The model under review builds one solid part; all positions refer to its coordinate system, in mm. A direction names the side the tool comes from. Round coordinates to 2 decimals unless told otherwise and drop trailing zeros. Write each loop counter-clockwise with the first axis right and the second up, starting at its lowest first coordinate (ties: lowest second). Pieces come first, ordered by that corner, then holes. Notation, with made-up numbers: (40.5, 66.5) -> (90.5, 66.5) arc R25 cw to (90.5, 100.5) -> close; hole circle Ø10 at (9.25, 9). An arc over 180 degrees is marked (long way). Answer in a Markdown table with one row per item. Add a question column.
```python
from build123d import *

# Parameters (mm, degrees)
SKETCH1_W           = 190.5
SKETCH1_H           = 6.35
BOSS_EXTRUDE1_DEPTH = 3.175
BOSS_EXTRUDE2_DEPTH = 3.175
LPATTERN1_COUNT     = 62
LPATTERN1_PITCH     = 2.54


with BuildPart() as part:
    # Sketch1 → Boss-Extrude1 (new body)
    with BuildSketch(Plane.XY):
        with Locations((95.25, 3.175)):
            Rectangle(SKETCH1_W, SKETCH1_H)
    extrude(amount=BOSS_EXTRUDE1_DEPTH)

    # Sketch2 → Boss-Extrude2 (add)
    with BuildSketch(Plane.XY.offset(3.175)):
        Polygon((165.1, 6.35), (163.83, 8.89), (162.56, 6.35), align=None)
    boss_extrude2 = extrude(amount=-BOSS_EXTRUDE2_DEPTH)

    # LPattern1: Boss-Extrude2 ×62
    with Locations(*[(-i * LPATTERN1_PITCH, 0, 0) for i in range(1, LPATTERN1_COUNT)]):
        add(boss_extrude2)


solid = part.part
```
1. Insertion check: pin 1 Ø1.5 at (x, z) = (46, 1.5) entering from +Y. The pin has a flat end and moves straight along its axis. Give the tip position at first contact, or say it passes through.
2. Tool access review of faces 1 (the flat face through (178, 6.35, 2)), 2 (the flat face through (94, 4, 0)), 3 (the flat face through (4, 6.35, 2)): name each direction out of +Z, -Z, +X, -X, +Y, -Y from which nothing blocks a thin tool from reaching the whole face with its end or side.
3. For L1, parallel to Y at x = 176.5, z = 0.9; L2, parallel to Y at x = 18.5, z = 2.85, list the stretches that pass through material, from the lowest coordinate up.
4. Add section A-A on x = 175.5. Write out the cut boundary in (y, z) (3 decimals).
Filled in:
| question | item | result |
|---|---|---|
| 1 | pin 1 | y = 8.41 |
| 2 | face 1 | +Z, -Z, +X, +Y |
| 2 | face 2 | -Z, +X, -X, +Y, -Y |
| 2 | face 3 | +Z, -Z, -X, +Y |
| 3 | L1 | 0 to 6.35 |
| 3 | L2 | 0 to 7.79 |
| 4 | outline | (0, 0) -> (6.35, 0) -> (6.35, 3.175) -> (0, 3.175) -> close |
